For this review, take the finished solid that the model builds, in its own axes (mm). Give positions to 0.01 mm unless a question says otherwise; leave off trailing zeros. Loops run counter-clockwise (first coordinate to the right, second up) from the corner with the lowest first, then second, coordinate; pieces in that order, holes last. Notation, with made-up numbers: (85, -34) - (113, -34) arc R27 cw to (113, -13) - close; hole circle Ø7 at (-35.75, 29.5). An arc over 180 degrees is marked (long way). Answer in a Markdown table with one row per item.
Autodesk Inventor part; units mm, degrees
ref_plane "YZ Plane" through (0, 0, 0) normal (1, 0, 0) x (0, 1, 0)
ref_plane "XZ Plane" through (0, 0, 0) normal (0, 1, 0) x (-1, 0, 0)
ref_plane "XY Plane" through (0, 0, 0) normal (0, 0, 1) x (1, 0, 0)
sketch "Base" plane through (0, 0, 0) normal (0, 0, 1) x (1, 0, 0)
  circle A0 centre (6.3437, -0.0043) radius 44.7044
  line L0 (-53.391, 43.8831) -> (3.4518, 87.3031)
  line L1 (3.4518, 87.3031) -> (126.7242, 46.1195)
  line L2 (21.9665, -51.542) -> (-11.8651, -109.4379)
  line L3 (134.9457, -71.4872) -> (143.2137, -54.1334)
  line L4 (44.7126, -49.2622) -> (124.7112, -76.8356)
  line L5 (44.7126, -49.2622) -> (21.9665, -51.542)
  line L6 (126.7242, 46.1195) -> (143.2137, -54.1334)
  line L7 (134.9457, -71.4872) -> (124.7112, -76.8356)
  line L8 (-30.3614, -103.0627) -> (-11.8651, -109.4379)
  line L9 (-30.3614, -103.0627) -> (-19.8027, -31.8971)
  line L10 (-54.6035, 18.8674) -> (-53.391, 43.8831)
  line L11 (-54.6035, 18.8674) -> (-19.8027, -31.8971)
  line L12 (-94.1669, 0) -> (182.7771, 0) construction
  circle A1 centre (6.3437, -0.0043) radius 3.175
  circle A2 centre (103.8642, -35.9814) radius 3.175
  line L13 (126.7242, 46.1195) -> (-19.8027, -31.8971) construction
  line L14 (3.4518, 87.3031) -> (33.3396, -50.4021) construction
  line L15 (-53.9972, 31.3753) -> (126.7242, 46.1195) construction
  line L16 (134.969, -4.007) -> (-37.2031, -6.5149) construction
  line L17 (-21.1132, -106.2503) -> (39.5241, 75.2519) construction
  line L18 (78.4642, -60.8955) -> (78.4642, 62.2425) construction
  line L19 (21.9665, -51.542) -> (126.7242, 46.1195) construction
  line L20 (0, 0) -> (-53.391, 43.8831) construction
  circle A3 centre (-20.3518, 21.9373) radius 3.175
  circle A4 centre (6.3437, -0.0043) radius 34.5555 construction
  circle A5 centre (-26.006, -12.1525) radius 3.175
  circle A6 centre (0.6895, -34.0941) radius 3.175
  circle A7 centre (33.0392, -21.9459) radius 3.175
  circle A8 centre (38.6934, 12.1439) radius 3.175
  circle A9 centre (11.9979, 34.0855) radius 3.175
  line L21 (113.2722, 38.9571) -> (102.0622, 32.9885) construction
  line L22 (111.78, 41.7596) -> (100.57, 35.791)
  line L23 (103.5543, 30.186) -> (114.7644, 36.1546)
  arc A10 (114.7644, 36.1546) -> (111.78, 41.7596) centre (113.2722, 38.9571) ccw
  arc A11 (100.57, 35.791) -> (103.5543, 30.186) centre (102.0622, 32.9885) ccw
  line L24 (119.5611, -4.2314) -> (106.8611, -4.2314) construction
  line L25 (119.5611, -1.0564) -> (106.8611, -1.0564)
  line L26 (106.8611, -7.4064) -> (119.5611, -7.4064)
  arc A12 (119.5611, -7.4064) -> (119.5611, -1.0564) centre (119.5611, -4.2314) ccw
  arc A13 (106.8611, -1.0564) -> (106.8611, -7.4064) centre (106.8611, -4.2314) ccw
  line L27 (6.6843, 72.4098) -> (9.378, 59.9988) construction
  line L28 (3.5815, 71.7364) -> (6.2752, 59.3254)
  line L29 (12.4807, 60.6722) -> (9.787, 73.0833)
  arc A14 (9.787, 73.0833) -> (3.5815, 71.7364) centre (6.6843, 72.4098) ccw
  arc A15 (6.2752, 59.3254) -> (12.4807, 60.6722) centre (9.378, 59.9988) ccw
  line L30 (-16.2839, -91.795) -> (-12.2597, -79.7494) construction
  line L31 (-13.2725, -92.801) -> (-9.2483, -80.7555)
  line L32 (-15.271, -78.7434) -> (-19.2953, -90.7889)
  arc A16 (-19.2953, -90.7889) -> (-13.2725, -92.801) centre (-16.2839, -91.795) ccw
  arc A17 (-9.2483, -80.7555) -> (-15.271, -78.7434) centre (-12.2597, -79.7494) ccw
  line L33 (78.4642, -44.7756) -> (78.4642, -32.0756) construction
  line L34 (75.2892, -44.7756) -> (75.2892, -32.0756)
  line L35 (81.6392, -32.0756) -> (81.6392, -44.7756)
  arc A18 (75.2892, -44.7756) -> (81.6392, -44.7756) centre (78.4642, -44.7756) ccw
  arc A19 (81.6392, -32.0756) -> (75.2892, -32.0756) centre (78.4642, -32.0756) ccw
  line L36 (-38.6678, 39.9478) -> (-26.0099, 40.9805) construction
  line L37 (-38.4097, 36.7833) -> (-25.7517, 37.816)
  line L38 (-26.2681, 44.145) -> (-38.926, 43.1123)
  arc A20 (-38.926, 43.1123) -> (-38.4097, 36.7833) centre (-38.6678, 39.9478) ccw
  arc A21 (-25.7517, 37.816) -> (-26.2681, 44.145) centre (-26.0099, 40.9805) ccw
  line L39 (45.5702, -29.5373) -> (54.8596, -20.8771) construction
  line L40 (47.7352, -31.8596) -> (57.0246, -23.1995)
  line L41 (52.6945, -18.5548) -> (43.4052, -27.2149)
  arc A22 (43.4052, -27.2149) -> (47.7352, -31.8596) centre (45.5702, -29.5373) ccw
  arc A23 (57.0246, -23.1995) -> (52.6945, -18.5548) centre (54.8596, -20.8771) ccw
  line L42 (-38.6678, 39.9478) -> (-53.391, 43.8831) construction
  circle A24 centre (122.4612, -51.192) radius 3
  point P0 (107.6672, 35.9728)
  point P1 (113.2111, -4.2314)
  point P2 (8.0311, 66.2043)
  point P3 (-14.2718, -85.7722)
  point P4 (78.4642, -38.4256)
  point P5 (-32.3389, 40.4642)
  point P6 (50.2149, -25.2072)
  dimension "d48" = 69.111
  dimension "d1" = 89.4088
  dimension "d2" = 55.568
  dimension "d3" = 37.094
  dimension "d4" = 120.3
  dimension "d5" = 81.561
  dimension "d6" = 160.982
  dimension "d7" = 133.392
  dimension "d8" = 143.066
  dimension "d9" = 145.185
  dimension "d10" = 124.151
  dimension "d11" = 130.15
  dimension "d12" = 142.793
  dimension "d13" = 117.814
  dimension "d14" = 19.5642
  dimension "d15" = 25.0158
  dimension "d16" = 71.529
  dimension "d17" = 61.5478
  dimension "d18" = 129.9699
  dimension "d19" = 101.6
  dimension "d20" = 19.2227
  dimension "d21" = 11.5477
  dimension "d22" = 84.6172
  dimension "d23" = 67.056
  dimension "d24" = 22.86
  dimension "d25" = 39.5986
  dimension "d26" = 71.1371
  dimension "d29" = 6.35
  dimension "d30" = 6.35
  dimension "d31" = 48.26
  dimension "d32" = 6.35
  dimension "d35" = 360
  dimension "d37" = 6.35
  dimension "d38" = 6.35
  dimension "d39" = 15.24
  dimension "d40" = 12.7
  dimension "d41" = 15.24
  dimension "d43" = 15.24
  dimension "d44" = 15.24
  dimension "d45" = 15.24
  dimension "d46" = 15.7016
  dimension "d49" = 140.583
  dimension "d50" = 4.2314
  dimension "d51" = 91.5631
  dimension "d52" = 12.1439
  dimension "d53" = 0
  dimension "d60" = 126.024
  dimension "d61" = 155.259
  dimension "d63" = 15.24
  dimension "d64" = 12.0647
  dimension "d67" = 25.4
  dimension "d68" = 31.75
  dimension "d69" = 6
  dimension "d70" = 20
  dimension "d71" = 20
extrude "Plate1" add sketch "Base" along normal blind 5 contours A0 L9 L11 | A0 L11 L10 L0 L1 L6 L3 L7 L4 L5 L2 L8 L9 | A5 picked at (-0.619, 18.5381)
fillet "OutsideFilletsFeature" radius 6.35 12 edges at (126.7242, 46.1195, 2.5) (3.4518, 87.3031, 2.5) (143.2137, -54.1334, 2.5) (134.9457, -71.4872, 2.5) (124.7112, -76.8356, 2.5) (-11.8651, -109.4379, 2.5) (44.7126, -49.2622, 2.5) (21.9665, -51.542, 2.5) (-30.3614, -103.0627, 2.5) (-19.8027, -31.8971, 2.5) (-54.6035, 18.8674, 2.5) (-53.391, 43.8831, 2.5)
sketch "HandleAttachment" plane through (0, 0, 0) normal (0, 0, -1) x (-1, 0, 0)
  circle A0 centre (-122.4612, -51.192) radius 3
  point P0 (0, 0)
equation "\"d41\" = d39"
equation "\"d43\" = d39"
equation "\"d44\" = d43"
equation "\"d45\" = d43"
equation "\"d47\" = Thickness"
properties part number "UpperLeg2"
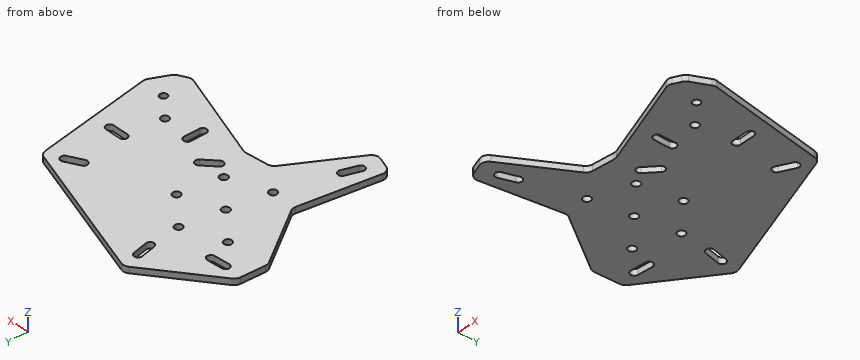
1. We need section A-A, the plane x = 69.5. Give the boundary of the cut face in (y, z).
Values:
| item | result |
|---|---|
| outline | (-57.81, 0) - (65.24, 0) - (65.24, 5) - (-57.81, 5) - close |
2. Clearance check with flat-ended pins moving along their axes: pin 1 (2 mm diameter, centred on x = 5, z = 2.5, fed in from -Y); pin 2 (1.5 mm diameter, centred on x = 111, z = 3, fed in from -Y); pin 3 (2 mm diameter, centred on x = 103, z = 1.5, fed in from +Y). State where each tip first meets the part, or that it passes through.
Values:
| item | result |
|---|---|
| pin 1 | stops at y = -82.29 |
| pin 2 | stops at y = -72.37 |
| pin 3 | stops at y = 54.38 |
3. Wall thickness on line 1 (Y direction, x = 109.5, z = 4.65); line 2 (X direction, y = 41, z = 3.65); line 3 (X direction, y = 19.5, z = 0.55): over which ranges is each line inside the solid? List them lowest first. Write a range as [from, to].
Values:
| item | result |
|---|---|
| line 1 | y = [-71.59, -7.41], [-1.06, 33.35], [40.55, 51.87] |
| line 2 | x = [-53.53, -41.66], [-22.83, 110.35], [115.7, 127.57] |
| line 3 | x = [-54.39, -22.39], [-18.32, 131.1] |
4. We need section B-B, the plane y = 53. Give the boundary of the cut face in (x, z).
Values:
| item | result |
|---|---|
| outline | (-41.46, 0) - (106.13, 0) - (106.13, 5) - (-41.46, 5) - close |
5. We need section C-C, the plane z = 1.7. Count the separate pieces of the cut face and the enclosed holes in it, and give its area (3 significant figures).
Values:
| item | result |
|---|---|
| separate pieces | 1 |
| enclosed holes | 15 |
| area | 22,500 mm^2 |
